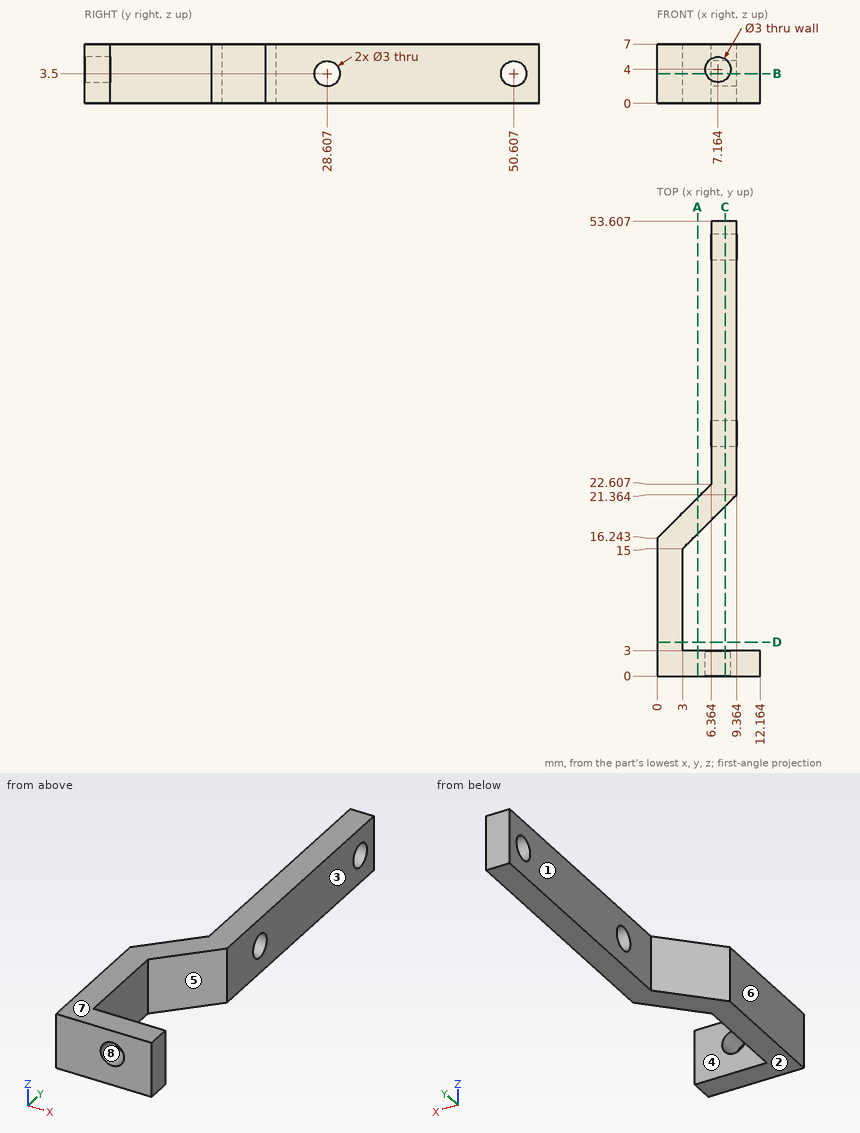
Here's the drawing with two shaded views (mm, measured from the low corner). I have some questions. A direction names the side the tool comes from. Round coordinates to 2 decimals unless told otherwise and drop trailing zeros. Loops run counter-clockwise (first coordinate to the right, second up) from the corner with the lowest first, then second, coordinate; pieces in that order, holes last. Notation, with made-up numbers: M 60.5,4 L 100.5,4 A16 cw 100.5,12 Z; hole C -6.75,77.5 d1. An arc over 180 degrees is marked long. Answer as CSV lines item,"result".
1) For pin 1 Ø4 at (y, z) = (28.61, 3.5) entering from -X; pin 2 Ø2.5 at (y, z) = (50.61, 3.5) entering from -X; pin 3 Ø4 at (x, y) = (4.5, 26) entering from -Z; pin 4 Ø2 at (y, z) = (12, 5) entering from +X, each with a flat end and sliding along its axis, tell me the tip position at first contact or that it passes through.
From the geometry:
pin 1,"x = 6.36"
pin 2,"through"
pin 3,"z = 0"
pin 4,"x = 3"
2) Imagine slicing it at B-B on z = 3.5. List the corners of the cut face in (x, y) for me, and give its area (3 significant figures).
From the geometry:
outline,"M 0,0 L 5.75,0 L 5.75,3 L 3,3 L 3,15 L 9.36,21.36 L 9.36,27.11 L 6.36,27.11 L 6.36,22.61 L 0,16.24 Z; M 6.36,30.11 L 9.36,30.11 L 9.36,49.11 L 6.36,49.11 Z; M 6.36,52.11 L 9.36,52.11 L 9.36,53.61 L 6.36,53.61 Z; M 8.58,0 L 12.16,0 L 12.16,3 L 8.58,3 Z"
area,"170 mm^2"
3) Imagine slicing it at A-A on x = 4.75. List the corners of the cut face in (y, z) for me, and give its area (3 significant figures).
From the geometry:
outline,"M 0,0 L 3,0 L 3,7 L 0,7 Z; M 16.75,0 L 20.99,0 L 20.99,7 L 16.75,7 Z"
area,"50.7 mm^2"
4) Imagine slicing it at C-C on x = 8. List the corners of the cut face in (y, z) for me (1 decimal).
From the geometry:
outline,"M 0,0 L 3,0 L 3,2.8 L 0,2.8 Z; M 0,5.2 L 3,5.2 L 3,7 L 0,7 Z; M 20,0 L 53.6,0 L 53.6,7 L 20,7 Z; hole C 28.6,3.5 d3; hole C 50.6,3.5 d3"
5) We'd pull the mould along X, two halves only. Please class the marked faces 5, 6, 7 and 8: released by +X, released by -X, zero draft, split by the parting line, or undercut.
From the geometry:
face 5,"released by +X"
face 6,"released by -X"
face 7,"zero draft"
face 8,"undercut"
6) Which directions (+Z, -Z, +X, -X, +Y, -Y) give clear straight access to the entire face, cutting with the end or side of a thin tool? Please do the marked faces 1, 2, 3 and 4.
From the geometry:
face 1,"+Z, -Z, -X, +Y"
face 2,"-Z, +X, -X, +Y, -Y"
face 3,"+Z, -Z, +X, +Y"
face 4,"+Z, -Z, +X"
7) Imagine slicing it at D-D on y = 4. List the corners of the cut face in (x, z) for me, and give its area (3 significant figures).
From the geometry:
outline,"M 0,0 L 3,0 L 3,7 L 0,7 Z"
area,"21.0 mm^2"
8) If I drill on probe 1 along X at (y, z) = (1.15, 4); probe 2 along X at (y, z) = (34.5, 1.75); probe 3 along Y at (x, z) = (9.5, 4), over which ranges is the centre line in solid material (lowest first)?
From the geometry:
probe 1,"0 to 5.66, 8.66 to 12.16"
probe 2,"6.36 to 9.36"
probe 3,"0 to 3"
